Answer from the drawing. Dimensions are ordinates in mm from the lowest x, y and z of the part. A direction names the side the tool comes from. Round coordinates to 2 decimals unless told otherwise and drop trailing zeros. Order: outer loops, then holes, each group sorted by start corner. A loop starts at its lowest first (then second) coordinate and runs counter-clockwise, first axis right, second up. Notation, with made-up numbers: M -20.5,84 L 20.5,84 A21 ccw 20.5,113 Z; hole C -33.75,0.25 d2. An arc over 180 degrees is marked long. Write item = value, one per line. Start each with the question number.
(1) Straight lines are drawn through the part: probe 1 along Z at (x, y) = (7.5, 0.8); probe 2 along X at (y, z) = (1.2, 15.5); probe 3 along Z at (x, y) = (5.75, 31). For each, find the intervals that lie inside material, in ascending order. Write a range as from..to.
(2) A cutting plane is placed at C-C, the plane x = 2. Determine the outline of the cut face in (y, z), and give its area (3 significant figures).
(3) A cutting plane is placed at A-A, the plane z = 15.5. Determine the outline of the cut face in (x, y).
(4) A cutting plane is placed at B-B, the plane x = 7.5. Determine the outline of the cut face in (y, z).
(5) Which of the six approach directions +Z, -Z, +X, -X, +Y, -Y give full straight-line access (tool end or side, diameter ignored) to the marked faces 1 and 2?
(6) Each of these flat-tipped pins is pushed along its axis until it touches: pin 1 (4.5 mm diameter, centred on x = 6, z = 8, fed in from +Y); pin 2 (7.5 mm diameter, centred on x = 5, y = 12.5, fed in from +Z). Where does it stop, or does it pass through?
(7) A cutting plane is placed at D-D, the plane y = 15. Determine the outline of the cut face in (x, z).
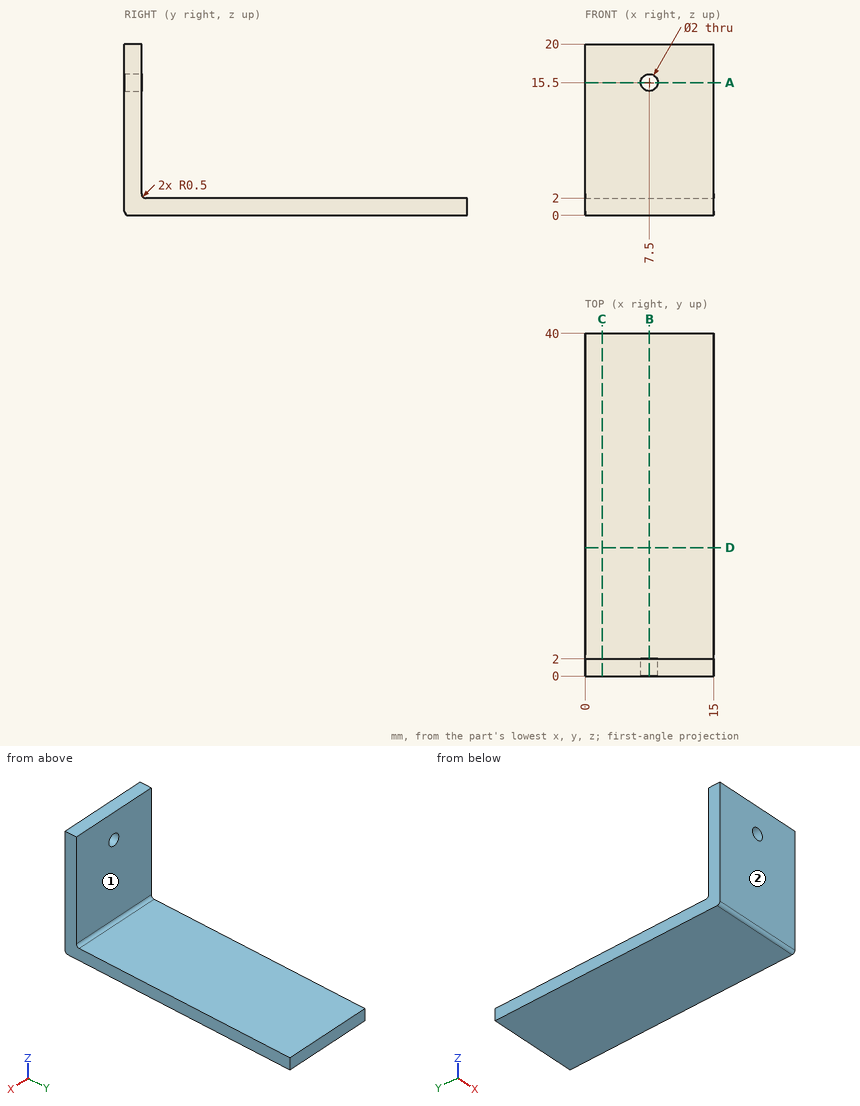
Reported:
q1.probe_1 = 0..14.5, 16.5..20
q1.probe_2 = 0..6.5, 8.5..15
q1.probe_3 = 0..2
q2.outline = M 0,0.5 A0.5 ccw 0.5,0 L 40,0 L 40,2 L 2.5,2 A0.5 cw 2,2.5 L 2,20 L 0,20 Z
q2.area = 116 mm²
q3.outline = M 0,0 L 6.5,0 L 6.5,2 L 0,2 Z; M 8.5,0 L 15,0 L 15,2 L 8.5,2 Z
q4.outline = M 0,0.5 A0.5 ccw 0.5,0 L 40,0 L 40,2 L 2.5,2 A0.5 cw 2,2.5 L 2,14.5 L 0,14.5 Z; M 0,16.5 L 2,16.5 L 2,20 L 0,20 Z
q5.face_1 = +Z, +X, -X, +Y
q5.face_2 = +Z, -Z, +X, -X, -Y
q6.pin_1 = 2
q6.pin_2 = 2
q7.outline = M 0,0 L 15,0 L 15,2 L 0,2 Z
